Autodesk Inventor part; units mm, degrees
ref_plane "YZ Plane" through (0, 0, 0) normal (1, 0, 0) x (0, 1, 0)
ref_plane "XZ Plane" through (0, 0, 0) normal (0, 1, 0) x (-1, 0, 0)
ref_plane "XY Plane" through (0, 0, 0) normal (0, 0, 1) x (1, 0, 0)
sketch "main profile" plane through (0, 0, 0) normal (0, 0, 1) x (1, 0, 0)
  line L0 (0, 0) -> (50.8, 0)
  line L1 (50.8, 0) -> (50.8, -12.7)
  line L2 (19.05, -31.75) -> (19.05, -44.45)
  line L3 (19.05, -44.45) -> (88.9, -44.45)
  line L4 (0, 0) -> (0, 88.9)
  line L5 (50.8, -12.7) -> (114.3, -12.7)
  line L6 (114.3, -12.7) -> (114.3, -25.4)
  line L7 (88.9, -44.45) -> (114.3, -25.4)
  line L8 (0, 88.9) -> (-6.35, 88.9)
  arc A0 (-6.35, 88.9) -> (-18.8698, 78.3317) centre (-6.35, 76.2) ccw
  line L9 (-18.8698, 78.3317) -> (-31.2996, 5.3292)
  arc A1 (-31.2996, 5.3292) -> (0, -31.75) centre (0, 0) ccw
  line L10 (19.05, -31.75) -> (0, -31.75)
  dimension "d8" = 50.8
  dimension "d9" = 12.7
  dimension "d11" = 69.85
  dimension "d15" = 114.3
  dimension "d16" = 12.7
  dimension "d18" = 44.45
  dimension "d20" = 19.05
  dimension "d41" = 12.7
  dimension "d42" = 31.75
  dimension "d44" = 31.75
  dimension "d45" = 120.65
  dimension "d56" = 6.35
  dimension "d64" = 114.3
extrude "FULL EXTRUSION" add sketch "main profile" along normal blind 76.2
sketch "Half Circle" plane through (0, 0, 0) normal (0, 1, 0) x (1, 0, 0)
  line L0 (50.8, 0) -> (50.8, -76.2)
  circle A0 centre (50.8, -38.1) radius 38.1
  point P0 (0, 0)
  dimension "d55" = 76.2
extrude "Half Circle Extrusion" add sketch "Half Circle" against normal up to surface (12.7 mm away)
sketch "Sketch6" plane through (0, 0, 76.2) normal (0, 1, 0) x (1, 0, 0)
  arc A0 (50.8, 0) -> (50.8, 76.2) centre (50.8, 38.1) ccw
  point P0 (0, 76.2)
hole "Hole2" at (50.8, 0, 38.1) direction (0, -1, 0) diameter 38.1 end through all
equation "\"d16\" = d9"
properties part number "ASN4-3-BK" material "Brass, Soft Yellow"
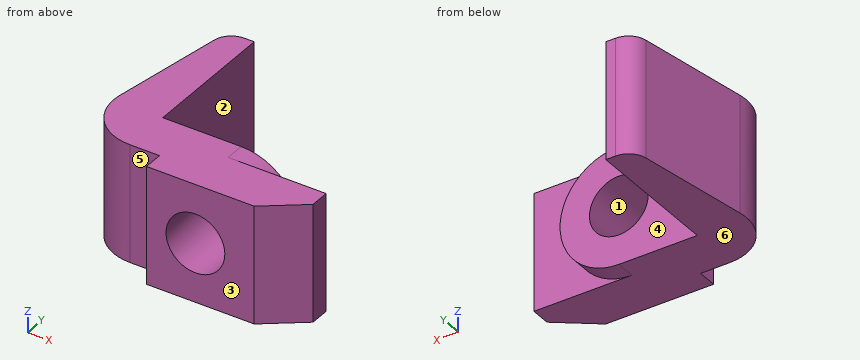
Verification items for the finished model (mm, model axes). Face numbers are marked on the shaded views. A direction names the side the tool comes from. Coordinates: 2 decimals unless noted, no trailing zeros. Write each loop counter-clockwise with the first axis right and the second up, starting at its lowest first coordinate (ties: lowest second). Pieces come first, ordered by that corner, then holes. Notation, with made-up numbers: M 40,10 L 59,10 A28 cw 59,41 Z; hole C -31.75,-2.75 d11. An arc over 180 degrees is marked long. Use a Markdown table: item, result.
Q1. Draft check along X on the marked faces 1, 2 and 3. Enter one of: +X half, -X half, draft (parallel to the pull), parting line (faces both ways), or undercut.
Reply:
| item | result |
|---|---|
| face 1 | undercut |
| face 2 | +X half |
| face 3 | draft |
Q2. Set-up check for the marked faces 4, 5 and 6: record each of +Z, -Z, +X, -X, +Y, -Y from which the full face is reachable in a straight line by a thin tool's end or side.
Reply:
| item | result |
|---|---|
| face 4 | +Z, -Z, +X, +Y |
| face 5 | +Z, -Z, -X, -Y |
| face 6 | -Z, +X, -X, +Y, -Y |
Q3. Sectioned sample at A-A, the plane z = 38.1. Record the boundary of the cut face in (x, y).
Reply:
| item | result |
|---|---|
| outline | M -31.3,5.33 A31.75 ccw 0,-31.75 L 19.05,-31.75 L 19.05,-44.45 L 31.75,-44.45 L 31.75,0 L 0,0 L 0,88.9 L -6.35,88.9 A12.7 ccw -18.87,78.33 Z; M 69.85,-44.45 L 88.9,-44.45 L 114.3,-25.4 L 114.3,-12.7 L 88.9,-12.7 L 88.9,0 L 69.85,0 Z |
Q4. Sectioned sample at B-B, the plane x = 66. Record the boundary of the cut face in (y, z).
Reply:
| item | result |
|---|---|
| outline | M -44.45,0 L -12.7,0 L -12.7,3.16 L 0,3.16 L 0,26.62 L -44.45,26.62 Z; M -44.45,49.58 L 0,49.58 L 0,73.04 L -12.7,73.04 L -12.7,76.2 L -44.45,76.2 Z |
Q5. Sectioned sample at D-D, the plane x = 27.5. Record the boundary of the cut face in (y, z).
Reply:
| item | result |
|---|---|
| outline | M -44.45,0 L 0,0 L 0,76.2 L -44.45,76.2 Z |
Q6. Sectioned sample at C-C, the plane z = 46. Record the boundary of the cut face in (x, y), plus the area to 3 significant figures.
Reply:
| item | result |
|---|---|
| outline | M -31.3,5.33 A31.75 ccw 0,-31.75 L 19.05,-31.75 L 19.05,-44.45 L 33.47,-44.45 L 33.47,0 L 0,0 L 0,88.9 L -6.35,88.9 A12.7 ccw -18.87,78.33 Z; M 68.13,-44.45 L 88.9,-44.45 L 114.3,-25.4 L 114.3,-12.7 L 88.07,-12.7 L 88.07,0 L 68.13,0 Z |
| area | 5,680 mm² |
Q7. Thickness scan on line 1 (Z direction, x = 50.8, y = -20.5); line 2 (X direction, y = -12, z = 38.1) (3 decimals); line 3 (X direction, y = -10, z = 38.1). Record the ranges inside material, lowest first.
Reply:
| item | result |
|---|---|
| line 1 | z = 0 to 19.05, 57.15 to 76.2 |
| line 2 | x = -29.395 to 31.75, 69.85 to 88.9 |
| line 3 | x = -30.13 to 31.75, 69.85 to 88.9 |
Q8. Go/stop test with flat-tipped pins: P1, Ø10, axis at y = -10, z = 67.5, coming from the -X side; P2, Ø1, axis at x = -7.5, z = 66, coming from the +Y side; P3, Ø1, axis at y = -28, z = 55.5, coming from the -X side. Record where each tip stops, or that it passes through.
Reply:
| item | result |
|---|---|
| P1 | stops at x = -31.35 |
| P2 | stops at y = 88.88 |
| P3 | stops at x = -15.87 |
